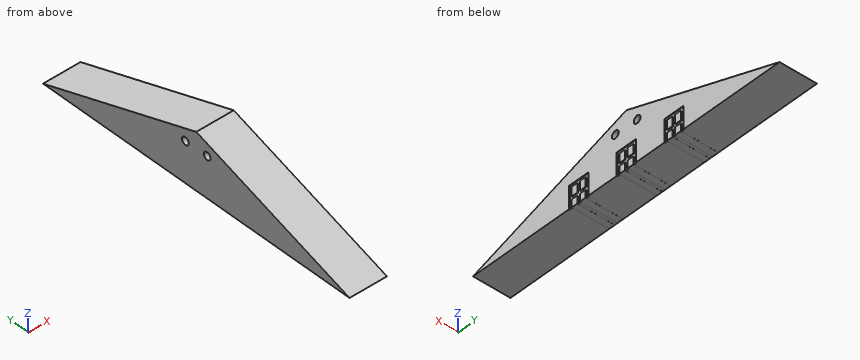
from build123d import *

# Parameters (mm, degrees)
F1_DEPTH  = 8
F3_DEPTH  = 621.7
F4_DEPTH  = 5.5
F7_DEPTH  = 5.5
F9_DEPTH  = 5.5
F11_DEPTH = 5.5
F13_DEPTH = 5.5
F15_DEPTH = 5.5
F17_DEPTH = 308.2
F18_DEPTH = 24
F20_DEPTH = 244.2
F21_DEPTH = 30.35
F22_R     = 2.5
F23_DEPTH = 0.5
F24_R     = 2.5
F25_DEPTH = 0.5
F26_R     = 2.5
F27_DEPTH = 0.5
F28_R     = 2.5
F29_DEPTH = 0.5
F30_W     = 14.1428571429
F30_H     = 18
F30_W_2   = 4.1785714286
F30_H_2   = 6.1071428571
F31_DEPTH = 0.5
F32_DEPTH = 25
F34_DEPTH = 8
F35_DEPTH = 0.5
F36_W     = 4.1785714286
F36_H     = 6.1071428571
F36_H_2   = 5.0357142857
F37_DEPTH = 24.5
F38_DEPTH = 25
F39_DEPTH = 1.05


# Not quite as in the source:
# - a feature of the source that left no trace in its solid (it failed there, or was rolled back) is left out


with BuildPart() as f1:
    # F0 (on Top) → F1 (new body)
    with BuildSketch(Plane.XY):
        Polygon((-327.3, 108.1424002851), (-327.3, -140.8575997149), (-102.6, -140.8575997149), (-102.6, -170.8575997149), (0, -170.8575997149), (0, -140.8575997149), (288.9, -140.8575997149), (288.9, 108.1424002851), (0, 108.1424002851), (0, 138.1424002851), (-102.6, 128.6424002851), (-102.6, 108.1424002851), align=None)
    extrude(amount=F1_DEPTH)

    # F2 (on face) → F3 (join)
    with BuildSketch(Plane.YZ.offset(288.9)):
        Polygon((-16.3575997149, 51.4532495908), (-146.3575997149, 8), (-140.8575997149, 8), (108.1424002851, 8), (113.6424002851, 8), align=None)
    extrude(amount=-F3_DEPTH)

    # F2 (on face) → F4 (join)
    with BuildSketch(Plane.YZ.offset(288.9)):
        Polygon((-16.3575997149, 51.4532495908), (-146.3575997149, 8), (113.6424002851, 8), align=None)
    extrude(amount=F4_DEPTH)

    # F5 (on face) → F7 (join)
    with BuildSketch(Plane.XZ.offset(170.8575997149)):
        Polygon((-51.3, 62.75), (-108.1, 8), (5.5, 8), align=None)
    extrude(amount=F7_DEPTH)

    # F8 (on face) → F9 (cut)
    with BuildSketch(Plane(origin=(-13.187163576, 142.4213666207, 0), x_dir=(-0.9957406741, -0.0921982106, 0), z_dir=(-0.0921982106, 0.9957406741, 0))):
        Polygon((91.8565413643, 4.3927081219), (38.2758658123, 55.8195932448), (-15.3048097397, 4.3927081219), align=None)
    extrude(amount=-F9_DEPTH, mode=Mode.SUBTRACT)

    # F10 (on face) → F11 (cut)
    with BuildSketch(Plane(origin=(-332.8, 0, 0), x_dir=(0, -1, 0), z_dir=(-1, 0, 0))):
        Polygon((144.6140170728, 2.7836871671), (16.3575997149, 45.6541342062), (-111.8988176431, 2.7836871671), align=None)
    extrude(amount=-F11_DEPTH, mode=Mode.SUBTRACT)

    # F12 (on face) → F13 (cut)
    with BuildSketch(Plane.YZ.offset(294.4)):
        Polygon((111.8988176431, 2.7836871671), (-16.3575997149, 45.6541342062), (-144.6140170728, 2.7836871671), align=None)
    extrude(amount=-F13_DEPTH, mode=Mode.SUBTRACT)

    # F14 (on face) → F15 (cut)
    with BuildSketch(Plane.XZ.offset(176.3575997149)):
        Polygon((1.6830285492, 4.0401099834), (-51.3, 55.1108989459), (-104.2830285492, 4.0401099834), align=None)
    extrude(amount=-F15_DEPTH, mode=Mode.SUBTRACT)

    # F16 (on face) → F17 (join)
    with BuildSketch(Plane.YZ.offset(294.4)):
        Polygon((-37.9123742622, 48.4659791319), (-36.6443145321, 44.6722981882), (-16.3575997149, 51.4532495908), (3.9291151024, 44.6722981882), (5.1971748325, 48.4659791319), (-16.3575997149, 55.670786811), align=None)
    extrude(amount=-F17_DEPTH)

    # F16 (on face) → F18 (cut)
    with BuildSketch(Plane.YZ.offset(294.4)):
        Polygon((-37.9123742622, 48.4659791319), (-36.6443145321, 44.6722981882), (-16.3575997149, 51.4532495908), (3.9291151024, 44.6722981882), (5.1971748325, 48.4659791319), (-16.3575997149, 55.670786811), align=None)
    extrude(amount=-F18_DEPTH, mode=Mode.SUBTRACT)

    # F19 (on face) → F20 (join)
    with BuildSketch(Plane(origin=(-332.8, 0, 0), x_dir=(0, -1, 0), z_dir=(-1, 0, 0))):
        Polygon((-5.1971748325, 48.4659791319), (-3.9291151024, 44.6722981882), (16.3575997149, 51.4532495908), (36.6443145321, 44.6722981882), (37.9123742622, 48.4659791319), (16.3575997149, 55.670786811), align=None)
    extrude(amount=-F20_DEPTH)

    # F19 (on face) → F21 (cut)
    with BuildSketch(Plane(origin=(-332.8, 0, 0), x_dir=(0, -1, 0), z_dir=(-1, 0, 0))):
        Polygon((-5.1971748325, 48.4659791319), (-3.9291151024, 44.6722981882), (16.3575997149, 51.4532495908), (36.6443145321, 44.6722981882), (37.9123742622, 48.4659791319), (16.3575997149, 55.670786811), align=None)
    extrude(amount=-F21_DEPTH, mode=Mode.SUBTRACT)

    # F22 (on face) → F23 (cut)
    with BuildSketch(Plane(origin=(-327.3, 0, 0), x_dir=(0, -1, 0), z_dir=(-1, 0, 0))):
        with Locations((8.3575997149, 35)):
            Circle(F22_R)
        with Locations((24.3575997149, 35)):
            Circle(F22_R)
    extrude(amount=-F23_DEPTH, mode=Mode.SUBTRACT)

    # F24 (on face) → F25 (cut)
    with BuildSketch(Plane.YZ.offset(288.9)):
        with Locations((-24.3575997149, 35)):
            Circle(F24_R)
        with Locations((-8.3575997149, 35)):
            Circle(F24_R)
    extrude(amount=-F25_DEPTH, mode=Mode.SUBTRACT)

    # F26 (on face) → F27 (cut)
    with BuildSketch(Plane.XZ.offset(170.8575997149)):
        with Locations((-59.3, 35)):
            Circle(F26_R)
        with Locations((-43.3, 35)):
            Circle(F26_R)
    extrude(amount=-F27_DEPTH, mode=Mode.SUBTRACT)

    # F28 (on face) → F29 (cut)
    with BuildSketch(Plane(origin=(-12.6822332802, 136.9681194259, 0), x_dir=(-0.9957406741, -0.0921982106, 0), z_dir=(-0.0921982106, 0.9957406741, 0))):
        with Locations((30.7829559704, 35)):
            Circle(F28_R)
        with Locations((46.7829559704, 35)):
            Circle(F28_R)
    extrude(amount=-F29_DEPTH, mode=Mode.SUBTRACT)

    # F30 (on face) → F31 (cut)
    with BuildSketch(Plane.YZ.offset(288.9)):
        with Locations((-16.3575997149, 14)):
            Rectangle(F30_W, F30_H)
        with Locations((-19.4111711434, 9.9821428571)):
            Rectangle(F30_W_2, F30_H_2, mode=Mode.SUBTRACT)
        with Locations((-13.3040282863, 9.9821428571)):
            Rectangle(F30_W_2, F30_H_2, mode=Mode.SUBTRACT)
        with Locations((-19.4111711434, 18.0178571429)):
            Rectangle(F30_W_2, F30_H_2, mode=Mode.SUBTRACT)
        with Locations((-13.3040282863, 18.0178571429)):
            Rectangle(F30_W_2, F30_H_2, mode=Mode.SUBTRACT)
        with Locations((18.6424002851, 14)):
            Rectangle(F30_W, F30_H)
        with Locations((15.5888288566, 9.9821428571)):
            Rectangle(F30_W_2, F30_H_2, mode=Mode.SUBTRACT)
        with Locations((21.6959717137, 9.9821428571)):
            Rectangle(F30_W_2, F30_H_2, mode=Mode.SUBTRACT)
        with Locations((15.5888288566, 18.0178571429)):
            Rectangle(F30_W_2, F30_H_2, mode=Mode.SUBTRACT)
        with Locations((21.6959717137, 18.0178571429)):
            Rectangle(F30_W_2, F30_H_2, mode=Mode.SUBTRACT)
        with Locations((-51.3575997149, 14)):
            Rectangle(F30_W, F30_H)
        with Locations((-54.4111711434, 9.9821428571)):
            Rectangle(F30_W_2, F30_H_2, mode=Mode.SUBTRACT)
        with Locations((-48.3040282863, 9.9821428571)):
            Rectangle(F30_W_2, F30_H_2, mode=Mode.SUBTRACT)
        with Locations((-54.4111711434, 18.0178571429)):
            Rectangle(F30_W_2, F30_H_2, mode=Mode.SUBTRACT)
        with Locations((-48.3040282863, 18.0178571429)):
            Rectangle(F30_W_2, F30_H_2, mode=Mode.SUBTRACT)
    extrude(amount=-F31_DEPTH, mode=Mode.SUBTRACT)


with BuildPart() as f32:
    # F32 (new): faces of the model
    f32_faces = [f1.part.faces().sort_by_distance(p)[0] for p in [
        (288.9, -16.3575997149, 2.5315074555),
        (288.4, -51.3575997149, 14),
        (288.4, -16.3575997149, 14),
        (288.4, 18.6424002851, 14),
    ]]
    extrude(f32_faces, amount=F32_DEPTH)

    # F34 (cut): a face of the model
    f34_faces = [f32.faces().sort_by_distance(p)[0] for p in [
        (301.4, -16.3575997149, 0),
    ]]
    extrude(f34_faces, amount=-F34_DEPTH, mode=Mode.SUBTRACT)

    # F35 (cut): faces of the model
    f35_faces = [f32.faces().sort_by_distance(p)[0] for p in [
        (288.4, 18.6424002851, 14),
        (288.4, -16.3575997149, 14),
        (288.4, -51.3575997149, 14),
    ]]
    extrude(f35_faces, amount=-F35_DEPTH, mode=Mode.SUBTRACT)

    # F36 (on face) → F37 (join)
    with BuildSketch(Plane(origin=(288.9, 0, 0), x_dir=(0, -1, 0), z_dir=(-1, 0, 0))):
        Polygon((61.9918890297, 25.6764385849), (-32.9998731613, 25.6764385849), (-32.9998731613, 8), (-23.785257428, 8), (-23.785257428, 13.0357142857), (-19.6066859994, 13.0357142857), (-19.6066859994, 8), (-17.6781145709, 8), (-17.6781145709, 13.0357142857), (-13.4995431423, 13.0357142857), (-13.4995431423, 8), (11.214742572, 8), (11.214742572, 13.0357142857), (15.3933140006, 13.0357142857), (15.3933140006, 8), (17.3218854291, 8), (17.3218854291, 13.0357142857), (21.5004568577, 13.0357142857), (21.5004568577, 8), (46.214742572, 8), (46.214742572, 13.0357142857), (50.3933140006, 13.0357142857), (50.3933140006, 8), (52.3218854291, 8), (52.3218854291, 13.0357142857), (56.5004568577, 13.0357142857), (56.5004568577, 8), (61.9918890297, 8), align=None)
        with Locations((-21.6959717137, 18.0178571429)):
            Rectangle(F36_W, F36_H, mode=Mode.SUBTRACT)
        with Locations((-15.5888288566, 18.0178571429)):
            Rectangle(F36_W, F36_H, mode=Mode.SUBTRACT)
        with Locations((13.3040282863, 18.0178571429)):
            Rectangle(F36_W, F36_H, mode=Mode.SUBTRACT)
        with Locations((19.4111711434, 18.0178571429)):
            Rectangle(F36_W, F36_H, mode=Mode.SUBTRACT)
        with Locations((48.3040282863, 18.0178571429)):
            Rectangle(F36_W, F36_H, mode=Mode.SUBTRACT)
        with Locations((54.4111711434, 18.0178571429)):
            Rectangle(F36_W, F36_H, mode=Mode.SUBTRACT)
        with Locations((-21.6959717137, 18.0178571429)):
            Rectangle(F36_W, F36_H)
        with Locations((-15.5888288566, 18.0178571429)):
            Rectangle(F36_W, F36_H)
        with Locations((-15.5888288566, 10.5178571429)):
            Rectangle(F36_W, F36_H_2)
        with Locations((-21.6959717137, 10.5178571429)):
            Rectangle(F36_W, F36_H_2)
        with Locations((13.3040282863, 18.0178571429)):
            Rectangle(F36_W, F36_H)
        with Locations((19.4111711434, 18.0178571429)):
            Rectangle(F36_W, F36_H)
        with Locations((19.4111711434, 10.5178571429)):
            Rectangle(F36_W, F36_H_2)
        with Locations((13.3040282863, 10.5178571429)):
            Rectangle(F36_W, F36_H_2)
        with Locations((48.3040282863, 18.0178571429)):
            Rectangle(F36_W, F36_H)
        with Locations((54.4111711434, 18.0178571429)):
            Rectangle(F36_W, F36_H)
        with Locations((54.4111711434, 10.5178571429)):
            Rectangle(F36_W, F36_H_2)
        with Locations((48.3040282863, 10.5178571429)):
            Rectangle(F36_W, F36_H_2)
    extrude(amount=-F37_DEPTH)

    # F30 (on face) → F38 (join)
    with BuildSketch(Plane.YZ.offset(288.9)):
        with Locations((21.6959717137, 18.0178571429)):
            Rectangle(F30_W_2, F30_H_2)
        with Locations((15.5888288566, 18.0178571429)):
            Rectangle(F30_W_2, F30_H_2)
        with Locations((15.5888288566, 9.9821428571)):
            Rectangle(F30_W_2, F30_H_2)
        with Locations((21.6959717137, 9.9821428571)):
            Rectangle(F30_W_2, F30_H_2)
        with Locations((-13.3040282863, 18.0178571429)):
            Rectangle(F30_W_2, F30_H_2)
        with Locations((-13.3040282863, 9.9821428571)):
            Rectangle(F30_W_2, F30_H_2)
        with Locations((-19.4111711434, 9.9821428571)):
            Rectangle(F30_W_2, F30_H_2)
        with Locations((-19.4111711434, 18.0178571429)):
            Rectangle(F30_W_2, F30_H_2)
        with Locations((-48.3040282863, 18.0178571429)):
            Rectangle(F30_W_2, F30_H_2)
        with Locations((-54.4111711434, 18.0178571429)):
            Rectangle(F30_W_2, F30_H_2)
        with Locations((-54.4111711434, 9.9821428571)):
            Rectangle(F30_W_2, F30_H_2)
        with Locations((-48.3040282863, 9.9821428571)):
            Rectangle(F30_W_2, F30_H_2)
    extrude(amount=F38_DEPTH)

    # F39 (cut): faces of the model
    f39_faces = [f32.faces().sort_by_distance(p)[0] for p in [
        (301.4, -54.4111711434, 6.9285714286),
        (301.4, -48.3040282863, 6.9285714286),
        (301.4, -19.4111711434, 6.9285714286),
        (301.4, -13.3040282863, 6.9285714286),
        (301.4, 15.5888288566, 6.9285714286),
        (301.4, 21.6959717137, 6.9285714286),
    ]]
    extrude(f39_faces, amount=-F39_DEPTH, mode=Mode.SUBTRACT)


solid = f32.part
Work out the finished part from the listing and answer in its coordinate system (mm). Coordinates: 2 decimals unless noted, no trailing zeros. Order: outer loops, then holes, each group sorted by start corner. A loop starts at its lowest first (then second) coordinate and runs counter-clockwise, first axis right, second up. Notation, with made-up numbers: (-16, 88.25) - (37, 88.25) arc R19 cw to (37, 109.25) - close; hole circle Ø7 at (-4.5, 24). An arc over 180 degrees is marked (long way). Put each result on its own line as item: value. Start each with the question number.
1) Find section D-D (y = 8). Give the vertices of the cut face in (x, z), plus the area to 3 significant figures.
2) Find section A-A (x = 297.5). State how many separate pieces and enclosed holes the cut face has, plus the area to 3 significant figures.
3) Flat-ended cylindrical pins translate along their axes: pin 1 (3 mm diameter, centred on x = 310.5, y = 47, fed in from -Z); pin 2 (5 mm diameter, centred on x = 299.5, y = -104.5, fed in from +Z); pin 3 (1 mm diameter, centred on x = 292, y = -95, fed in from +Z). Find the tip coordinate at first contact, or state that the pin passes through.
4) Find section B-B (z = 35). Give the vertices of the cut face in (x, y), plus the area to 3 significant figures.
5) Find the intervals of material crossed by line 1 (X direction, y = -50, z = 13.5); line 2 (Z direction, x = 307.75, y = -25); line 3 (Z direction, x = 290, y = -85.5), in increasing order. Write a range as from..to.
6) Find section C-C (y = 46.5). Give the vertices of the cut face in (x, z), plus the area to 3 significant figures.
Results list:
1. outline: (288.9, 8) - (313.9, 8) - (313.9, 37.51) - (288.9, 37.51) - close
1. area: 738 mm^2
2. separate pieces: 1
2. enclosed holes: 2
2. area: 4,200 mm^2
3. pin 1: stops at z = 8
3. pin 2: stops at z = 17.03
3. pin 3: stops at z = 19.53
4. outline: (288.9, -48.23) - (313.9, -48.23) - (313.9, -26.86) - (288.9, -26.86) - close; (288.9, -21.86) - (313.9, -21.86) - (313.9, -10.86) - (288.9, -10.86) - close; (288.9, -5.86) - (313.9, -5.86) - (313.9, 15.52) - (288.9, 15.52) - close
4. area: 1,340 mm^2
5. line 1: x = 288.9..313.4
5. line 2: z = 8..32.58, 37.42..42.77
5. line 3: z = 8..22.54
6. outline: (288.9, 8) - (313.9, 8) - (313.9, 24.64) - (288.9, 24.64) - close
6. area: 416 mm^2
